Job drawing, mm, ordinate dimensions from the low corner. One solid piece. Coordinates: 2 decimals unless noted, no trailing zeros. Loops run counter-clockwise (first coordinate to the right, second up) from the corner with the lowest first, then second, coordinate; pieces in that order, holes last. Notation, with made-up numbers: (-24, -21.5) - (0, -21.5) arc R22 cw to (0, 7.5) - close; hole circle Ø8 at (28, -10). An arc over 180 degrees is marked (long way). Use a Markdown table: item, result. Add a question column.
1. Band-saw the part on C-C, the plane x = 5.25. Count the separate pieces of the cut face and the enclosed holes in it, plus the area to 3 significant figures.
2. Drop flat-ended pins along their axis: pin 1 (0.9 mm diameter, centred on x = 6.5, y = 5, fed in from +Z); pin 2 (2 mm diameter, centred on x = 7, z = 13, fed in from -Y); pin 3 (2 mm diameter, centred on y = 3, z = 35.5, fed in from -X). Give the stop position or say it passes through.
3. Pull direction Z, two halves, no side cores. Call the marked faces 1, 2 and 3: pulls with the +Z half, pulls with the -Z half, needs draft (parallel to the pull), parting line crosses it, or undercut.
4. Band-saw the part on B-B, the plane z = 35.5. Give the cut face in (x, y).
5. Band-saw the part on D-D, the plane x = 10. Give the cut face in (y, z).
6. Wall check: probe 1 along Z at (x, y) = (2.75, 1); probe 2 along X at (y, z) = (5.75, 21); probe 3 along Z at (x, y) = (10, 6). Give the ranges that are in metal, low to high. Write a range as [from, to].
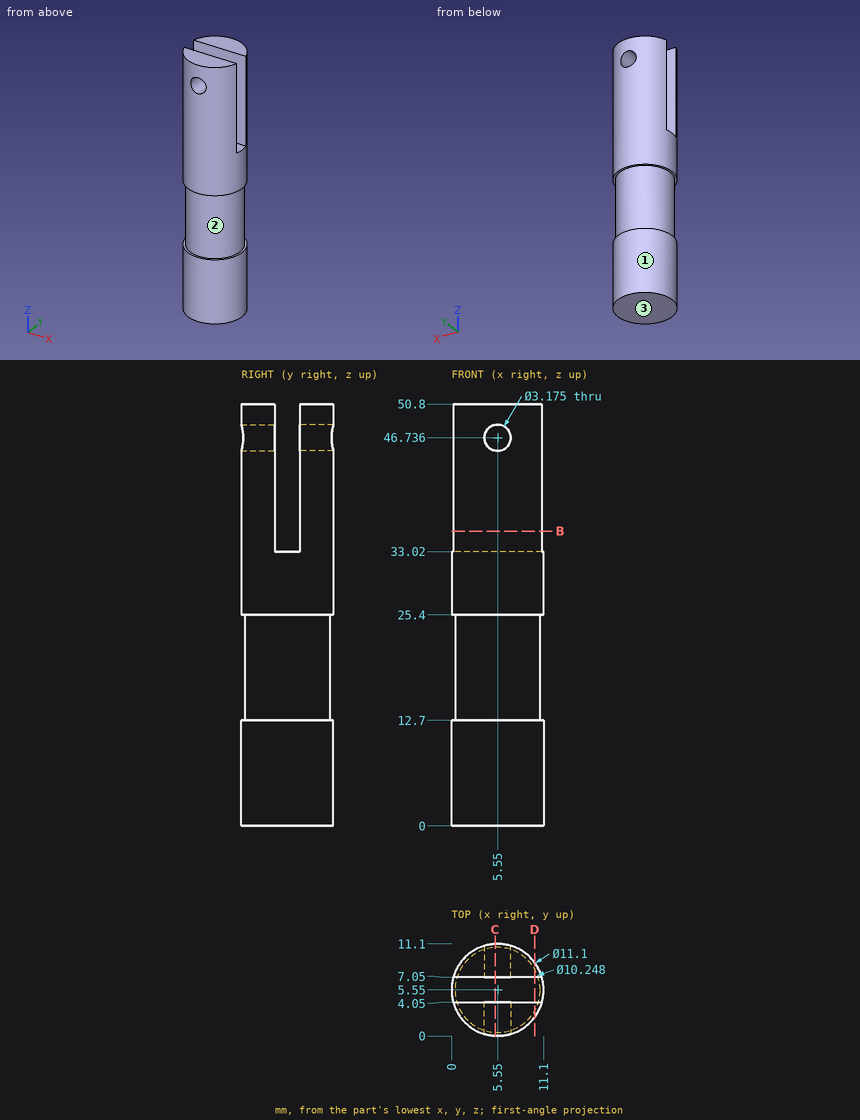
Geometry check:
| question | item | result |
|---|---|---|
| 1 | separate pieces | 3 |
| 1 | enclosed holes | 0 |
| 1 | area | 474 mm^2 |
| 2 | pin 1 | stops at z = 33.02 |
| 2 | pin 2 | stops at y = 0.02 |
| 2 | pin 3 | stops at x = 0.22 |
| 3 | face 1 | needs draft |
| 3 | face 2 | undercut |
| 3 | face 3 | pulls with the -Z half |
| 4 | outline | (0.21, 4.05) arc R5.55 ccw to (10.89, 4.05) - close; (0.21, 7.05) - (10.89, 7.05) arc R5.55 ccw to start |
| 5 | outline | (2.23, 0) - (8.87, 0) - (8.87, 12.7) - (8.09, 12.7) - (8.09, 25.4) - (8.87, 25.4) - (8.87, 50.8) - (7.05, 50.8) - (7.05, 33.02) - (4.05, 33.02) - (4.05, 50.8) - (2.23, 50.8) - (2.23, 25.4) - (3.01, 25.4) - (3.01, 12.7) - (2.23, 12.7) - close |
| 6 | probe 1 | z = [0, 12.7], [25.4, 50.8] |
| 6 | probe 2 | x = [0.43, 10.67] |
| 6 | probe 3 | z = [0, 33.02] |
